Design review of the part built by this model. Coordinates are the model's own, in mm. Face numbers are marked on the shaded views. A direction names the side the tool comes from. Coordinates: 2 decimals unless noted, no trailing zeros. Loops run counter-clockwise (first coordinate to the right, second up) from the corner with the lowest first, then second, coordinate; pieces in that order, holes last. Notation, with made-up numbers: (16.25, 39) -> (43.25, 39) arc R20 cw to (43.25, 46) -> close; hole circle Ø11 at (56.25, 12.25). An arc over 180 degrees is marked (long way). Use a Markdown table: item, result. Add a question column.
Q1. For probe 1 along X at (y, z) = (0, -0.75); probe 2 along Z at (x, y) = (-2, 4.5), list the stretches that pass through material, from the lowest coordinate up.
Q2. Take a section at A-A on x = 0. Write out the cut boundary in (y, z) (3 decimals).
Q3. Take a section at B-B on z = 3.5. Write out the cut boundary in (x, y), plus the area to 3 significant figures.
Q4. Take a section at C-C on z = 0.5. Write out the cut boundary in (x, y), plus the area to 3 significant figures.
Q5. Draft analysis for pull direction Y (two halves, no side actions). For the marked faces 3, 4 and 5, state which applies: pulls with the +Y half, pulls with the -Y half, needs draft (parallel to the pull), parting line crosses it, or undercut.
Q6. Clearance check with flat-ended pins moving along their axes: pin 1 Ø1.2 at (x, y) = (7.5, 0) entering from -Z; pin 2 Ø2 at (y, z) = (2, 3) entering from -X; pin 3 Ø5.5 at (x, y) = (-1.5, -1) entering from -Z. State where each tip first meets the part, or that it passes through.
Q7. For the marked faces 1 and 2, list the 3-axis set-ups (+Z, -Z, +X, -X, +Y, -Y) from which the entire face can be reached by the end or side of a thin tool; tool diameter is ignored.
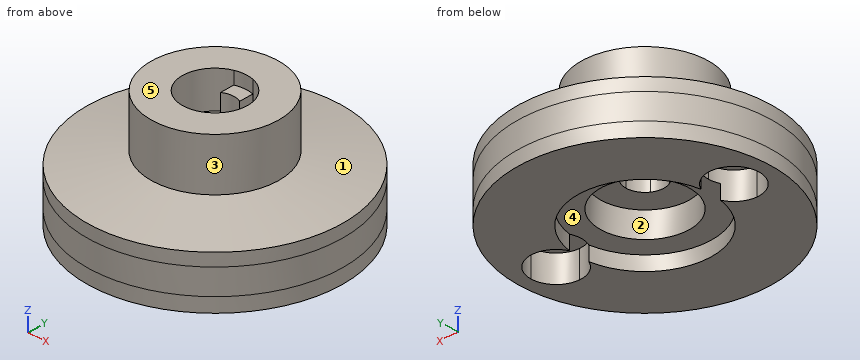
from build123d import *

# Parameters (mm, degrees)
F0_R      = 5
F1_DEPTH  = 6
F2_DEPTH  = 5
F3_DEPTH  = 3.1
F6_R      = 10
F6_R_2    = 3.5
F7_DEPTH  = 2
F8_R      = 10
F8_R_2    = 5.25
F9_DEPTH  = 1.125
F11_DEPTH = 2.125


with BuildPart() as f1:
    # F0 (on Top) → F1 (new body)
    with BuildSketch(Plane.XY):
        Circle(F0_R)
        with BuildLine():
            ThreePointArc((0.75, 2.4372115214), (2.0512191497, 1.5149257408), (2.55, 0))
            ThreePointArc((2.55, 0), (2.0512191497, -1.5149257408), (0.75, -2.4372115214))
            ThreePointArc((0.75, -2.4372115214), (0, -2.55), (-0.75, -2.4372115214))
            ThreePointArc((-0.75, -2.4372115214), (-2.55, 0), (-0.75, 2.4372115214))
            ThreePointArc((-0.75, 2.4372115214), (0, 2.55), (0.75, 2.4372115214))
        make_face(mode=Mode.SUBTRACT)
    extrude(amount=F1_DEPTH)

    # F0 (on Top) → F2 (join)
    with BuildSketch(Plane.XY):
        with BuildLine():
            Line((0.75, 1.2990381057), (0.75, 2.4372115214))
            ThreePointArc((0.75, 2.4372115214), (0, 2.55), (-0.75, 2.4372115214))
            Line((-0.75, 2.4372115214), (-0.75, 1.2990381057))
            ThreePointArc((-0.75, 1.2990381057), (0, 1.5), (0.75, 1.2990381057))
        make_face()
        with BuildLine():
            ThreePointArc((-0.75, -2.4372115214), (0, -2.55), (0.75, -2.4372115214))
            Line((0.75, -2.4372115214), (0.75, -1.2990381057))
            ThreePointArc((0.75, -1.2990381057), (0, -1.5), (-0.75, -1.2990381057))
            Line((-0.75, -1.2990381057), (-0.75, -2.4372115214))
        make_face()
    extrude(amount=F2_DEPTH)

    # F0 (on Top) → F3 (join)
    with BuildSketch(Plane.XY):
        with BuildLine():
            Line((-0.75, 1.2990381057), (-0.75, 2.4372115214))
            ThreePointArc((-0.75, 2.4372115214), (-2.55, 0), (-0.75, -2.4372115214))
            Line((-0.75, -2.4372115214), (-0.75, -1.2990381057))
            ThreePointArc((-0.75, -1.2990381057), (-1.5, 0), (-0.75, 1.2990381057))
        make_face()
        with BuildLine():
            ThreePointArc((0.75, -2.4372115214), (2.0512191497, -1.5149257408), (2.55, 0))
            ThreePointArc((2.55, 0), (2.0512191497, 1.5149257408), (0.75, 2.4372115214))
            Line((0.75, 2.4372115214), (0.75, 1.2990381057))
            ThreePointArc((0.75, 1.2990381057), (1.2990381057, 0.75), (1.5, 0))
            ThreePointArc((1.5, 0), (1.2990381057, -0.75), (0.75, -1.2990381057))
            Line((0.75, -1.2990381057), (0.75, -2.4372115214))
        make_face()
    extrude(amount=F3_DEPTH)

    # F4 (on Front) → F5 (revolve)
    with BuildSketch(Plane.XZ):
        Polygon((-10, 0), (-4, 0), (-4, 2), (-4.5, 2), (-10, 1), align=None)
    revolve(axis=Axis((0, 0, 1.2425027974), (0, 0, 1)))

    # F6 (on face) → F7 (join)
    with BuildSketch(Plane(origin=(0, 0, 0), x_dir=(1, 0, 0), z_dir=(0, 0, -1))):
        Circle(F6_R)
        Circle(F6_R_2, mode=Mode.SUBTRACT)
    extrude(amount=F7_DEPTH)

    # F8 (on face) → F9 (join)
    with BuildSketch(Plane(origin=(0, 0, -2), x_dir=(1, 0, 0), z_dir=(0, 0, -1))):
        Circle(F8_R)
        Circle(F8_R_2, mode=Mode.SUBTRACT)
    extrude(amount=F9_DEPTH)

    # F10 (on face) → F11 (cut)
    with BuildSketch(Plane(origin=(0, 0, -3.125), x_dir=(1, 0, 0), z_dir=(0, 0, -1))):
        with BuildLine():
            ThreePointArc((-7, -2), (-5.5857864376, -1.4142135624), (-5, 0))
            ThreePointArc((-5, 0), (-5.5857864376, 1.4142135624), (-7, 2))
            ThreePointArc((-7, 2), (-9, 0), (-7, -2))
        make_face()
        with BuildLine():
            ThreePointArc((7, -2), (8.4142135624, -1.4142135624), (9, 0))
            ThreePointArc((9, 0), (8.4142135624, 1.4142135624), (7, 2))
            ThreePointArc((7, 2), (5, 0), (7, -2))
        make_face()
    extrude(amount=-F11_DEPTH, mode=Mode.SUBTRACT)


solid = f1.part
Answer list:
| question | item | result |
|---|---|---|
| 1 | probe 1 | -10 to -3.5, 3.5 to 10 |
| 1 | probe 2 | -2 to 6 |
| 2 | outline | (-10, -3.125) -> (-5.25, -3.125) -> (-5.25, -2) -> (-3.5, -2) -> (-3.5, 0) -> (-1.5, 0) -> (-1.5, 5) -> (-2.55, 5) -> (-2.55, 6) -> (-5, 6) -> (-5, 1.909) -> (-10, 1) -> close; (1.5, 0) -> (3.5, 0) -> (3.5, -2) -> (5.25, -2) -> (5.25, -3.125) -> (10, -3.125) -> (10, 1) -> (5, 1.909) -> (5, 6) -> (2.55, 6) -> (2.55, 5) -> (1.5, 5) -> close |
| 3 | outline | circle Ø10 at (0, 0); hole (-0.75, -2.44) -> (-0.75, -1.3) arc R1.5 ccw to (0.75, -1.3) -> (0.75, -2.44) arc R2.55 ccw to (0.75, 2.44) -> (0.75, 1.3) arc R1.5 ccw to (-0.75, 1.3) -> (-0.75, 2.44) arc R2.55 ccw to start |
| 3 | area | 61.3 mm² |
| 4 | outline | circle Ø20 at (0, 0); hole circle Ø3 at (0, 0) |
| 4 | area | 307 mm² |
| 5 | face 3 | parting line crosses it |
| 5 | face 4 | undercut |
| 5 | face 5 | needs draft |
| 6 | pin 1 | z = -1 |
| 6 | pin 2 | x = -4.9 |
| 6 | pin 3 | z = -2 |
| 7 | face 1 | +Z |
| 7 | face 2 | -Z |
